Input: dimensioned drawing with shaded views. Units: mm. Origin: part minimum x, y, z. A direction names the side the tool comes from. Give positions to 0.01 mm unless a question says otherwise; leave off trailing zeros. Write each loop counter-clockwise with the first axis right and the second up, starting at its lowest first coordinate (ties: lowest second). Pieces come first, ordered by that corner, then holes. Notation, with made-up numbers: (14.5, 17.25) -> (59.5, 17.25) arc R6 cw to (59.5, 24.25) -> close; hole circle Ø7 at (-27.5, 36). An arc over 180 degrees is marked (long way). Answer as a JSON object with one key per item and string values.
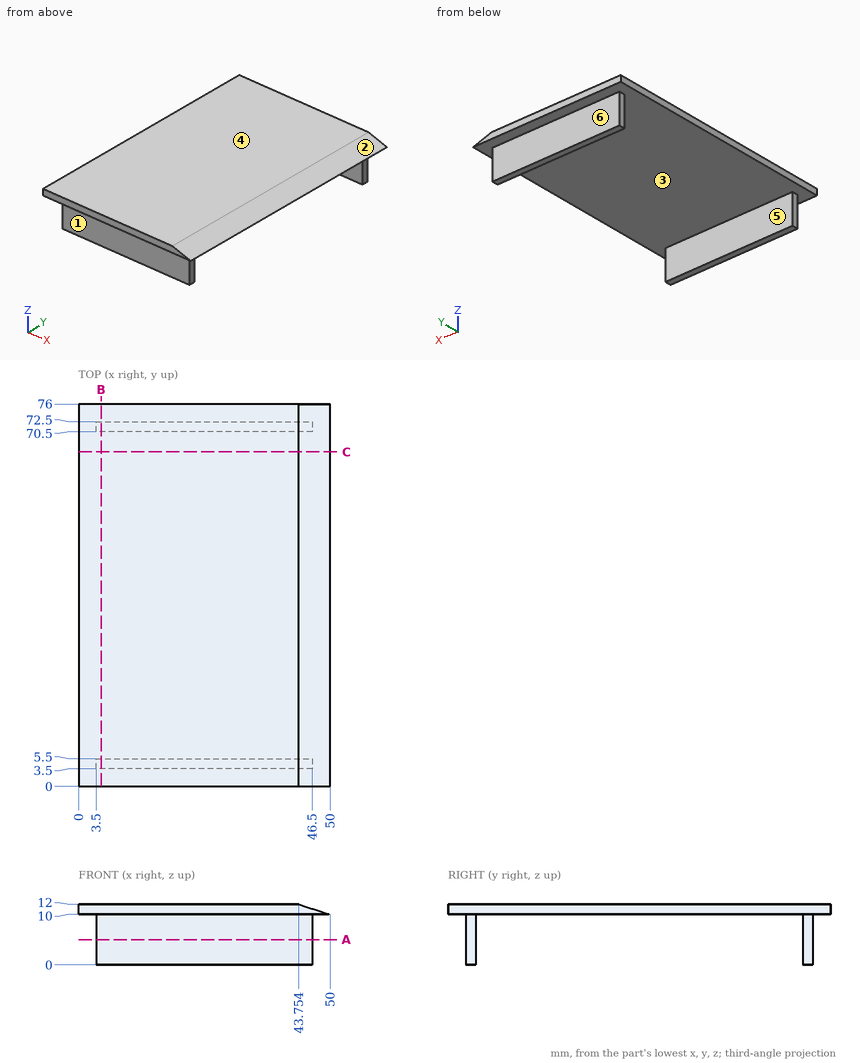
Q1. Cut plane A-A (z = 5). Return the cut outline in (x, y), and give its area (3 significant figures).
Values:
{"outline": "(3.5, 3.5) -> (46.5, 3.5) -> (46.5, 5.5) -> (3.5, 5.5) -> close; (3.5, 70.5) -> (46.5, 70.5) -> (46.5, 72.5) -> (3.5, 72.5) -> close", "area": "172 mm²"}
Q2. Material intervals for L1, parallel to Y at x = 7, z = 9.75; L2, parallel to Z at x = 7.5, y = 24, sorted ascending. Write a range as from..to.
Values:
{"L1": "3.5..5.5, 70.5..72.5", "L2": "10..12"}
Q3. Mould query, pull axis Y, two halves, no side actions, for the marked faces 1, 2 and 3. Classes: pulls with the +Y half, pulls with the -Y half, needs draft (parallel to the pull), parting line crosses it, or undercut.
Values:
{"face 1": "pulls with the -Y half", "face 2": "needs draft", "face 3": "undercut"}
Q4. Cut plane C-C (y = 66.5). Return the cut outline in (x, z).
Values:
{"outline": "(0, 10) -> (50, 10) -> (43.75, 12) -> (0, 12) -> close"}
Q5. First-contact query: P1, Ø2, axis at x = 33, y = 41.5, coming from the -Z side; P2, Ø3, axis at x = 23, z = 8, coming from the +Y side; P3, Ø1.6, axis at y = 4.5, z = 7, coming from the +X side. Flat tips, straight axial feed; report the tip coordinate or a pass-through.
Values:
{"P1": "z = 10", "P2": "y = 72.5", "P3": "x = 46.5"}
Q6. Set-up query: the marked faces 4, 5 and 6. Return all of +Z, -Z, +X, -X, +Y, -Y with unobstructed straight access to the full face (end or side cutting, diameter ignored); none if empty.
Values:
{"face 4": "+Z, +X, -X, +Y, -Y", "face 5": "-Z, +X, -X", "face 6": "-Z, +X, -X, +Y"}
Q7. Cut plane B-B (x = 4.5). Return the cut outline in (y, z).
Values:
{"outline": "(0, 10) -> (3.5, 10) -> (3.5, 0) -> (5.5, 0) -> (5.5, 10) -> (70.5, 10) -> (70.5, 0) -> (72.5, 0) -> (72.5, 10) -> (76, 10) -> (76, 12) -> (0, 12) -> close"}
